from build123d import *

# Parameters (mm, degrees)
CROQUIS1_R              = 42.5
SALIENTE_EXTRUIR1_DEPTH = 5
SALIENTE_EXTRUIR2_DEPTH = 2
CROQUIS3_R              = 1.7
CORTAR_EXTRUIR1_DEPTH   = 21
CROQUIS4_R              = 2.95
CORTAR_EXTRUIR2_DEPTH   = 3


with BuildPart() as part:
    # Croquis1 → Saliente-Extruir1 (new body)
    with BuildSketch(Plane(origin=(0, 0, 0), x_dir=(1, 0, 0), z_dir=(0, 1, 0))):
        with BuildLine():
            ThreePointArc((39.782879484, 48.85), (0, 63), (-39.782879484, 48.85))
            ThreePointArc((-39.782879484, 48.85), (-32.82545617, 87.047566078), (-47.293763221, 123.077107909))
            ThreePointArc((-47.293763221, 123.077107909), (0, 220), (47.293763221, 123.077107909))
            ThreePointArc((47.293763221, 123.077107909), (32.82545617, 87.047566078), (39.782879484, 48.85))
        make_face()
        with Locations((0, 160)):
            Circle(CROQUIS1_R, mode=Mode.SUBTRACT)
    extrude(amount=SALIENTE_EXTRUIR1_DEPTH)

    # Croquis2 → Saliente-Extruir2 (add)
    with BuildSketch(Plane(origin=(0, 5, 0), x_dir=(1, 0, 0), z_dir=(0, 1, 0))):
        with BuildLine():
            Line((5, 205), (-5, 205))
            Line((-5, 205), (-5, 219.791303716))
            ThreePointArc((-5, 219.791303716), (0, 220), (5, 219.791303716))
            Line((5, 219.791303716), (5, 205))
        make_face()
    extrude(amount=SALIENTE_EXTRUIR2_DEPTH)

    # Croquis3 → Cortar-Extruir1 (cut)
    with BuildSketch(Plane(origin=(0, 7, 0), x_dir=(1, 0, 0), z_dir=(0, 1, 0))):
        with Locations((0, 215)):
            Circle(CROQUIS3_R)
        with Locations((-28.5, 86.5)):
            Circle(CROQUIS3_R)
        with Locations((-28.5, 73.5)):
            Circle(CROQUIS3_R)
        with Locations((28.5, 73.5)):
            Circle(CROQUIS3_R)
        with Locations((28.5, 86.5)):
            Circle(CROQUIS3_R)
    extrude(amount=-CORTAR_EXTRUIR1_DEPTH, mode=Mode.SUBTRACT)

    # Croquis4 → Cortar-Extruir2 (cut)
    with BuildSketch(Plane.XZ):
        with Locations((0, -215)):
            Circle(CROQUIS4_R)
    extrude(amount=-CORTAR_EXTRUIR2_DEPTH, mode=Mode.SUBTRACT)


solid = part.part
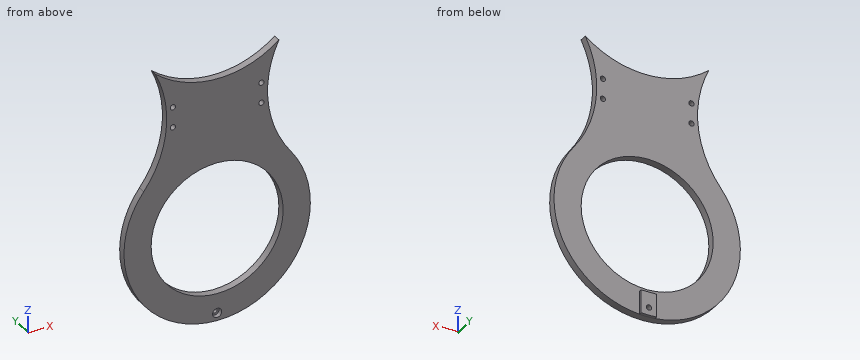
Can you work these out from the model? Positions are in its coordinate system, mm. Give positions to 0.01 mm unless a question says otherwise; leave off trailing zeros. Order: outer loops, then holes, each group sorted by start corner. A loop starts at its lowest first (then second) coordinate and runs counter-clockwise, first axis right, second up. Notation, with made-up numbers: M 84,24 L 122,24 A30 cw 122,46 Z; hole C 31.25,-3 d1. An arc over 180 degrees is marked long. Use one line per item in the form item = value. Start each with the question number.
Item 1: If we section it at B-B (z = -160): Write out the boundary of the cut face in (x, y), then the cut area to 3 significant figures.
Item 2: If I drill on line 1 along Z through (x, y) = (-38, 3.5); line 2 along Z through (x, y) = (29, 4.5); line 3 along Y through (x, z) = (17, -95.5), over which ranges is the centre line in solid material (lowest first)?
Item 3: If we section it at D-D (z = -73.5): Write out the boundary of the cut face in (x, y).
Item 4: If we section it at C-C (y = 1.5): Write out the boundary of the cut face in (x, z).
Item 5: If we section it at A-A (x = 0): Write out the boundary of the cut face in (y, z), then the cut area to 3 significant figures.
Item 6: Will these pins go through, and if not, where does the flat tip stop? pin 1 Ø1.6 at (y, z) = (6.5, -216) entering from -X; pin 2 Ø1.6 at (x, y) = (-2, 6.5) entering from +Z; pin 3 Ø1 at (x, y) = (38, 2.5) entering from -Z.
Outcome:
q1.outline = M -60,0 L -42.5,0 L -42.5,5 L -60,5 Z; M 42.5,0 L 60,0 L 60,5 L 42.5,5 Z
q1.area = 175 mm2
q2.line_1 = -206.43 to -179.03, -140.97 to -107.27, -52.73 to -50.25
q2.line_2 = -212.53 to -191.07, -128.93 to -88.12, -84.88 to -75.12, -71.88 to -55.93
q2.line_3 = 0 to 5
q3.outline = M -32.77,0 L -30.2,0 L -30.2,5 L -32.77,5 Z; M -26.8,0 L 26.8,0 L 26.8,5 L -26.8,5 Z; M 30.2,0 L 32.77,0 L 32.77,5 L 30.2,5 Z
q4.outline = M -47.29,-123.08 A60 ccw long 47.29,-123.08 A70 cw 39.78,-48.85 A63 cw -39.78,-48.85 A70 cw Z; hole C 0,-160 d85; hole C -28.5,-86.5 d3.4; hole C -28.5,-73.5 d3.4; hole C 0,-215 d5.9; hole C 28.5,-86.5 d3.4; hole C 28.5,-73.5 d3.4
q5.outline = M 0,-220 L 7,-220 L 7,-216.7 L 3,-216.7 L 3,-217.95 L 0,-217.95 Z; M 0,-212.05 L 3,-212.05 L 3,-213.3 L 7,-213.3 L 7,-205 L 5,-205 L 5,-202.5 L 0,-202.5 Z; M 0,-117.5 L 5,-117.5 L 5,-63 L 0,-63 Z
q5.area = 359 mm2
q6.pin_1 = -5
q6.pin_2 = -205
q6.pin_3 = -206.84
